Geometry: final body of the model. Coordinates: model frame, mm. Face numbers are marked on the shaded views. A direction names the side the tool comes from. Give positions to 0.01 mm unless a question says otherwise; leave off trailing zeros. Write each loop counter-clockwise with the first axis right and the second up, starting at its lowest first coordinate (ties: lowest second). Pieces come first, ordered by that corner, then holes.
Q1. Pin query (flat end, axial travel): pin 1 Ø10 at (y, z) = (32.5, -22) entering from +X; pin 2 Ø20 at (x, y) = (1.5, 14) entering from +Z; pin 3 Ø12 at (x, z) = (52, -9.5) entering from +Y; pin 4 Ø1.8 at (x, z) = (-66, -14.75) entering from -Y. Return the tip coordinate at first contact, or that it passes through.
Q2. Mould query, pull axis Z, two halves, no side actions, for the marked faces 1, 2 and 3. Classes: +Z half, -Z half, draft (parallel to the pull), parting line (faces both ways), or undercut.
Q3. Section B-B (y = 32). Return the cut outline in (x, z).
Q4. Section C-C (z = -68.75). Return the cut outline in (x, y), plus the area to 3 significant figures.
Q5. Reachability of the marked faces 4, 5, 6 and 7 from +Z, -Z, +X, -X, +Y, -Y: full face, straight path, thin tool, end or side. Return the list, or none.
Q6. Line query: line 1 (Y direction, x = 47.5, z = -1); line 2 (X direction, y = 22, z = -49); line 3 (X direction, y = 1.25, z = 21.25). Output: solid intervals per line, ascending.
Q7. Section A-A (x = -32). Return the cut outline in (y, z), plus the area to 3 significant figures.
Q8. Section D-D (x = 35). Return the cut outline in (y, z).
from build123d import *

# Parameters (mm, degrees)
SKETCH1_R           = 1.5
BOSS_EXTRUDE1_DEPTH = 2.8
BOSS_EXTRUDE2_DEPTH = 38
CUT_EXTRUDE1_REACH  = 136.827
SKETCH4_W           = 16
SKETCH4_H           = 20
BOSS_EXTRUDE3_DEPTH = 18
CHAMFER1_SIZE       = 18
SKETCH5_R           = 6.5
BOSS_EXTRUDE4_DEPTH = 1
SKETCH6_R           = 3
BOSS_EXTRUDE5_DEPTH = 20
BOSS_EXTRUDE6_DEPTH = 15
SKETCH8_R           = 4
BOSS_EXTRUDE7_DEPTH = 10


with BuildPart() as part:
    # Sketch1 → Boss-Extrude1 (new body)
    with BuildSketch(Plane(origin=(0, 0, 0), x_dir=(1, 0, 0), z_dir=(0, 1, 0))):
        Polygon((56, 23.75), (56, 64.75), (-76, 64.75), (-76, -64.75), (76, -64.75), (76, 23.75), align=None)
        with Locations(Location((66, -21.25, 0), (0, 0, 270))):
            Circle(SKETCH1_R, mode=Mode.SUBTRACT)
        with Locations(Location((-66, 14.75, 0), (0, 0, 270))):
            Circle(SKETCH1_R, mode=Mode.SUBTRACT)
        with Locations(Location((-46, 51.75, 0), (0, 0, 270))):
            Circle(SKETCH1_R, mode=Mode.SUBTRACT)
        with Locations(Location((46, 51.75, 0), (0, 0, 270))):
            Circle(SKETCH1_R, mode=Mode.SUBTRACT)
    extrude(amount=BOSS_EXTRUDE1_DEPTH)

    # Sketch2 → Boss-Extrude2 (add)
    with BuildSketch(Plane(origin=(0, 2.8, 0), x_dir=(1, 0, 0), z_dir=(0, 1, 0))):
        Polygon((-35, 59.75), (-35, -5.25), (30, -5.25), (30, 9.75), (40, 9.75), (40, 59.75), align=None)
    extrude(amount=BOSS_EXTRUDE2_DEPTH)

    # Sketch3 → Cut-Extrude1 (cut, up to next)
    with BuildSketch(Plane.ZY.offset(35), mode=Mode.PRIVATE) as cut_extrude1_sk1:
        Polygon((5.25, 20.8), (-9.75, 35.8), (-21.75, 40.8), (5.25, 40.8), align=None)
    cut_extrude1_tool1 = extrude(cut_extrude1_sk1.sketch, amount=-CUT_EXTRUDE1_REACH, mode=Mode.PRIVATE) & part.part
    add(cut_extrude1_tool1.solids().sort_by_distance((-35, 34.535632, -2.543103))[0], mode=Mode.SUBTRACT)

    # Sketch4 → Boss-Extrude3 (add)
    with BuildSketch(Plane(origin=(0, 0, -59.75), x_dir=(-1, 0, 0), z_dir=(0, 0, -1))):
        with Locations((-20, 31.8)):
            Rectangle(SKETCH4_W, SKETCH4_H)
    extrude(amount=BOSS_EXTRUDE3_DEPTH)

    # Chamfer1
    chamfer1_edges = [part.edges().sort_by_distance(p)[0] for p in [
        (20, 21.8, -77.75),
    ]]
    chamfer(chamfer1_edges, length=CHAMFER1_SIZE - 0.0001)  # a hair under: the kernel refuses the full size

    # Sketch5 → Boss-Extrude4 (add)
    with BuildSketch(Plane(origin=(0, 41.8, 0), x_dir=(1, 0, 0), z_dir=(0, 1, 0))):
        with Locations(Location((20, 68.75, 0), (0, 0, 270))):
            Circle(SKETCH5_R)
    extrude(amount=BOSS_EXTRUDE4_DEPTH)

    # Sketch6 → Boss-Extrude5 (add)
    with BuildSketch(Plane(origin=(0, 42.8, 0), x_dir=(1, 0, 0), z_dir=(0, 1, 0))):
        with Locations(Location((20, 68.75, 0), (0, 0, 270))):
            Circle(SKETCH6_R)
    extrude(amount=BOSS_EXTRUDE5_DEPTH)

    # Sketch7 → Boss-Extrude6 (add)
    with BuildSketch(Plane.XY.offset(-24.75)):
        Polygon((26, 40.8), (4, 40.8), (7.5, 46.862177826), (22.5, 46.862177826), align=None)
    extrude(amount=-BOSS_EXTRUDE6_DEPTH)

    # Sketch8 → Boss-Extrude7 (add)
    with BuildSketch(Plane(origin=(0, 46.862177826, 0), x_dir=(1, 0, 0), z_dir=(0, 1, 0))):
        with Locations(Location((15, 32.25, 0), (0, 0, 270))):
            Circle(SKETCH8_R)
    extrude(amount=BOSS_EXTRUDE7_DEPTH)


solid = part.part
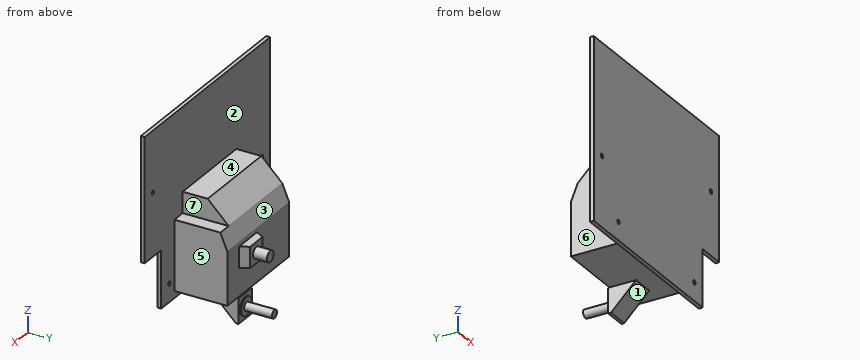
Computed:
1. pin 1: stops at x = 40
1. pin 2: stops at z = 5.25
1. pin 3: stops at y = 2.8
1. pin 4: passes through
2. face 1: -Z half
2. face 2: draft
2. face 3: +Z half
3. outline: (-35, -59.75) - (12, -59.75) - (12, -69.95) - (28, -69.95) - (28, -59.75) - (40, -59.75) - (40, -9.75) - (30, -9.75) - (30, -5.95) - (-35, -5.95) - close
4. outline: (12, 30.8) - (28, 30.8) - (28, 41.8) - (26.5, 41.8) - (26.5, 42.8) - (23, 42.8) - (23, 62.8) - (17, 62.8) - (17, 42.8) - (13.5, 42.8) - (13.5, 41.8) - (12, 41.8) - close
4. area: 309 mm2
5. face 4: +Z, +X, -X, +Y
5. face 5: +Z, -Z, +X, +Y
5. face 6: +Z, -Z, -X, +Y
5. face 7: +Z, +X, +Y
6. line 1: y = 0 to 2.8
6. line 2: x = -35 to 40
6. line 3: x = -76 to 64.5, 67.5 to 76
7. outline: (0, -64.75) - (2.8, -64.75) - (2.8, -59.75) - (40.8, -59.75) - (40.8, -21.75) - (35.8, -9.75) - (20.8, 5.25) - (2.8, 5.25) - (2.8, 64.75) - (0, 64.75) - close
7. area: 2,620 mm2
8. outline: (0, -64.75) - (2.8, -64.75) - (2.8, -59.75) - (40.8, -59.75) - (40.8, -21.75) - (35.8, -9.75) - (2.8, -9.75) - (2.8, 64.75) - (0, 64.75) - close
